Design review of the part built by this model. Coordinates are the model's own, in mm. Face numbers are marked on the shaded views. A direction names the side the tool comes from. Give positions to 0.01 mm unless a question says otherwise; leave off trailing zeros. Write each loop counter-clockwise with the first axis right and the second up, starting at its lowest first coordinate (ties: lowest second). Pieces come first, ordered by that corner, then holes. Notation, with made-up numbers: (30, 16) -> (86, 16) arc R35 ccw to (86, 51) -> close; hole circle Ø9 at (-30.5, 11). An arc over 180 degrees is marked (long way). Write each question's results on one line, items separated by ' | '. Start each with the question number.
(1) For the marked faces 1, 2, 3 and 4, list the 3-axis set-ups (+Z, -Z, +X, -X, +Y, -Y) from which the entire face can be reached by the end or side of a thin tool; tool diameter is ignored.
(2) Clearance check with flat-ended pins moving along their axes: pin 1 (4 mm diameter, centred on x = -25, z = 5.5, fed in from +Y); pin 2 (10 mm diameter, centred on x = 13.5, z = 3, fed in from +Y); pin 3 (5 mm diameter, centred on y = 6.5, z = 33.5, fed in from -X). State where each tip first meets the part, or that it passes through.
(3) Mouldability with a two-part tool opening along Z and no side actions: class the marked faces 5, 6, 7 and 8 as released by +Z, released by -Z, zero draft, split by the parting line, or undercut.
(4) Take a section at B-B (y = 17). State the section outline as (x, z) points.
(5) Take a section at A-A (z = 0). State the section outline as (x, y) points, plus the area to 3 significant figures.
(6) To check wall thickness, follow probe 1 along X at (y, z) = (38, -5); probe 2 along Z at (x, y) = (24, 38); probe 3 along Z at (x, y) = (-14.5, 17). State the ranges of each line that lie inside material, in increasing order.
(7) Take a section at C-C (x = 32). State the section outline as (y, z) points.
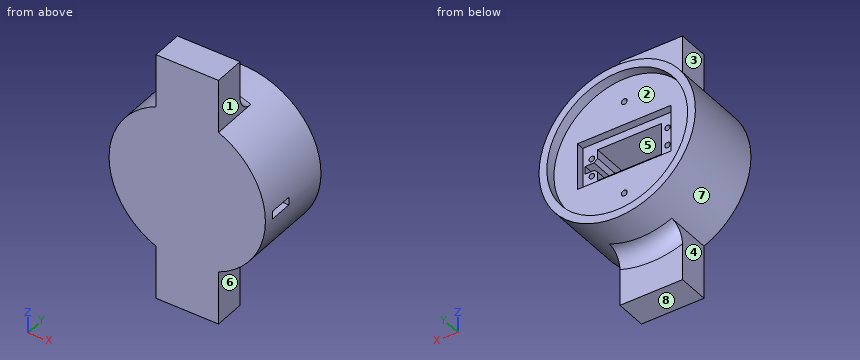
from build123d import *

# Parameters (mm, degrees)
ESQUISSE1_R             = 50
BOSS_EXTRU_1_DEPTH      = 45
ESQUISSE2_W             = 60
ESQUISSE2_H             = 30
ENL_V_MAT_EXTRU_2_DEPTH = 5
ENL_V_MAT_EXTRU_4_DEPTH = 38.2
ESQUISSE2_4_R           = 50
ESQUISSE2_4_R_2         = 45
BOSS_EXTRU_2_DEPTH      = 6.6
ESQUISSE2_5_R           = 1.75
ENL_V_MAT_EXTRU_5_DEPTH = 10
ESQUISSE3_R             = 1.85
ENL_V_MAT_EXTRU_6_DEPTH = 10
BOSS_EXTRU_3_START      = -13
ESQUISSE4_W             = 40
ESQUISSE4_H             = 20
BOSS_EXTRU_3_DEPTH      = 43
CONG_1_R                = 10
ESQUISSE5_W             = 5
ESQUISSE5_H             = 15
ENL_V_MAT_EXTRU_7_DEPTH = 124.388856936


with BuildPart() as part:
    # Esquisse1 → Boss.-Extru.1 (new body)
    with BuildSketch(Plane(origin=(0, 0, 0), x_dir=(1, 0, 0), z_dir=(0, 1, 0))):
        with Locations(Location((0, 0, 0), (0, 0, 90))):
            Circle(ESQUISSE1_R)
    extrude(amount=BOSS_EXTRU_1_DEPTH)

    # Esquisse2 → Enl_v. mat.-Extru.2 (cut)
    with BuildSketch(Plane(origin=(0, 45, 0), x_dir=(1, 0, 0), z_dir=(0, 1, 0))):
        Rectangle(ESQUISSE2_W, ESQUISSE2_H)
    extrude(amount=-ENL_V_MAT_EXTRU_2_DEPTH, mode=Mode.SUBTRACT)

    # Esquisse2_3 → Enl_v. mat.-Extru.4 (cut)
    with BuildSketch(Plane(origin=(0, 45, 0), x_dir=(1, 0, 0), z_dir=(0, 1, 0))):
        Polygon((-20.5, 10.1), (20.5, 10.1), (20.5, 4.5), (22.736067977, 2.5), (28.5, 2.5), (28.5, -2.5), (22.736067977, -2.5), (20.5, -4.5), (20.5, -10.1), (-20.5, -10.1), align=None)
    extrude(amount=-ENL_V_MAT_EXTRU_4_DEPTH, mode=Mode.SUBTRACT)

    # Esquisse2_4 → Boss.-Extru.2 (add)
    with BuildSketch(Plane(origin=(0, 45, 0), x_dir=(1, 0, 0), z_dir=(0, 1, 0))):
        with Locations(Location((0, 0, 0), (0, 0, 90))):
            Circle(ESQUISSE2_4_R)
        with Locations(Location((0, 0, 0), (0, 0, 270))):
            Circle(ESQUISSE2_4_R_2, mode=Mode.SUBTRACT)
    extrude(amount=BOSS_EXTRU_2_DEPTH)

    # Esquisse2_5 → Enl_v. mat.-Extru.5 (cut)
    with BuildSketch(Plane(origin=(0, 45, 0), x_dir=(1, 0, 0), z_dir=(0, 1, 0))):
        with Locations(Location((24.2, -5.65, 0), (0, 0, 270))):
            Circle(ESQUISSE2_5_R)
        with Locations(Location((24.2, 5.65, 0), (0, 0, 270))):
            Circle(ESQUISSE2_5_R)
        with Locations(Location((-24.2, 5.65, 0), (0, 0, 270))):
            Circle(ESQUISSE2_5_R)
        with Locations(Location((-24.2, -5.65, 0), (0, 0, 270))):
            Circle(ESQUISSE2_5_R)
    extrude(amount=-ENL_V_MAT_EXTRU_5_DEPTH, mode=Mode.SUBTRACT)

    # Esquisse3 → Enl_v. mat.-Extru.6 (cut)
    with BuildSketch(Plane(origin=(0, 45, 0), x_dir=(1, 0, 0), z_dir=(0, 1, 0))):
        with Locations(Location((0, 30, 0), (0, 0, 270))):
            Circle(ESQUISSE3_R)
        with Locations(Location((0, -30, 0), (0, 0, 90))):
            Circle(ESQUISSE3_R)
    extrude(amount=-ENL_V_MAT_EXTRU_6_DEPTH, mode=Mode.SUBTRACT)

    # Esquisse4 → Boss.-Extru.3 (add)
    with BuildSketch(Plane.XY.offset(50).offset(BOSS_EXTRU_3_START)):
        with Locations((0, 10)):
            Rectangle(ESQUISSE4_W, ESQUISSE4_H)
    boss_extru_3 = extrude(amount=BOSS_EXTRU_3_DEPTH)

    # Sym_trie1: Boss.-Extru.3 across plane
    add(boss_extru_3.mirror(Plane.XY))

    # Cong_1
    cong_1_edges = [part.edges().sort_by_distance(p)[0] for p in [
        (-10.215482184, 20, -48.945315647),
        (0, 20, 50),
    ]]
    fillet(cong_1_edges, radius=CONG_1_R)

    # Esquisse5 → Enl_v. mat.-Extru.7 (cut, through all)
    with BuildSketch(Plane.ZY.offset(-28.5)):
        with Locations((0, 14.3)):
            Rectangle(ESQUISSE5_W, ESQUISSE5_H)
    extrude(amount=-ENL_V_MAT_EXTRU_7_DEPTH, mode=Mode.SUBTRACT)


solid = part.part
Report:
1) face 1: +Z, +X, +Y, -Y | face 2: +Y | face 3: +Z, -X, +Y, -Y | face 4: -Z, -X, +Y, -Y
2) pin 1: y = 40 | pin 2: y = 6.8 | pin 3: x = -39.23
3) face 5: undercut | face 6: zero draft | face 7: split by the parting line | face 8: released by -Z
4) outline: (-20.5, -10.1) -> (-20.5, 10.1) -> (20.5, 10.1) -> (20.5, 4.5) -> (22.74, 2.5) -> (49.94, 2.5) arc R50 ccw to (20, 45.83) -> (20, 80) -> (-20, 80) -> (-20, 45.83) arc R50 ccw to (-20, -45.83) -> (-20, -80) -> (20, -80) -> (20, -45.83) arc R50 ccw to (49.94, -2.5) -> (22.74, -2.5) -> (20.5, -4.5) -> (20.5, -10.1) -> close
5) outline: (-50, 0) -> (50, 0) -> (50, 6.8) -> (-20.5, 6.8) -> (-20.5, 40) -> (-30, 40) -> (-30, 45) -> (-45, 45) -> (-45, 51.6) -> (-50, 51.6) -> close; (28.5, 21.8) -> (50, 21.8) -> (50, 51.6) -> (45, 51.6) -> (45, 45) -> (30, 45) -> (30, 40) -> (28.5, 40) -> close | area: 2,320 mm2
6) probe 1: -49.75 to -25.82, -22.58 to -20.5, 20.5 to 22.58, 25.82 to 49.75 | probe 2: -43.86 to -7.39, -3.91 to -2.5, 2.5 to 3.91, 7.39 to 43.86 | probe 3: -80 to -10.1, 10.1 to 80
7) outline: (0, -38.42) -> (51.6, -38.42) -> (51.6, -31.64) -> (45, -31.64) -> (45, 31.64) -> (51.6, 31.64) -> (51.6, 38.42) -> (0, 38.42) -> close; hole (6.8, -2.5) -> (21.8, -2.5) -> (21.8, 2.5) -> (6.8, 2.5) -> close
